Job drawing, mm, ordinate dimensions from the low corner. One solid piece. Coordinates: 2 decimals unless noted, no trailing zeros. Loops run counter-clockwise (first coordinate to the right, second up) from the corner with the lowest first, then second, coordinate; pieces in that order, holes last. Notation, with made-up numbers: (9, 22.25) -> (19, 22.25) arc R32 cw to (19, 49.25) -> close; hole circle Ø11 at (65, -31). An arc over 180 degrees is marked (long way). Use one line per item in the form item = value. Start each with the question number.
(1) Band-saw the part on C-C on y = 1.4. Give the cut face in (x, z).
(2) Band-saw the part on B-B on x = 17.7. Give the cut face in (y, z).
(3) Drill centre lines: L1, parallel to X at y = 1.55, z = 10.5; L2, parallel to Y at x = 16, z = 17.25; L3, parallel to X at y = 2.95, z = 11.5. Where is each one in solid material? Low to high. Write a range as [from, to].
(4) Pin check, flat tips, straight feed: P1, Ø1.8, axis at x = 10.5, z = 17.7, coming from the +Y side; P2, Ø1.5, axis at x = 7, y = 2.5, coming from the -Z side; P3, Ø2, axis at y = 4, z = 12.5, coming from the -X side. Stop position of each tip, or through.
(5) Mould opens along X. For the marked faces 1, 2 and 3 say: +X half, -X half, draft (parallel to the pull), parting line (faces both ways), or undercut.
(6) Band-saw the part on A-A on z = 10.5. Give the cut face in (x, y), then the cut area to 3 significant figures.
(7) Band-saw the part on D-D on z = 3.25. Give the cut face in (x, y), then the cut area to 3 significant figures.
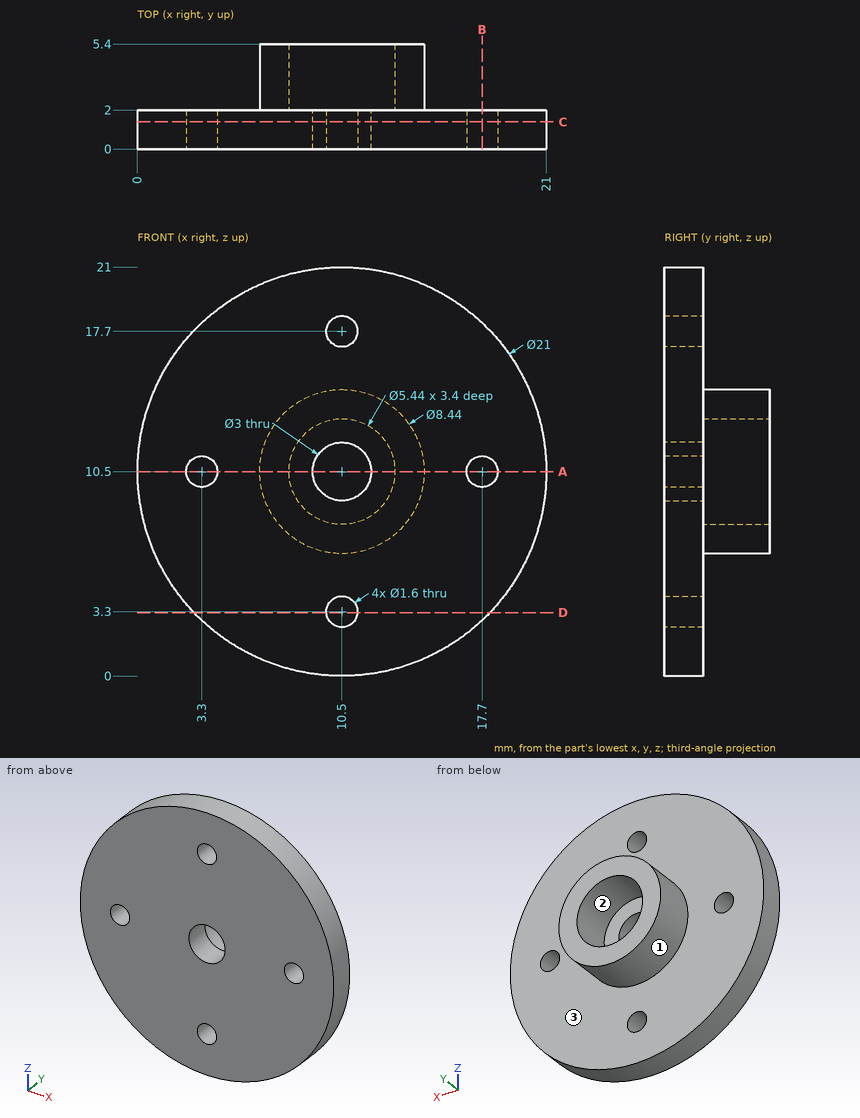
A:
q1.outline = circle Ø21 at (10.5, 10.5); hole circle Ø1.6 at (3.3, 10.5); hole circle Ø3 at (10.5, 10.5); hole circle Ø1.6 at (10.5, 3.3); hole circle Ø1.6 at (10.5, 17.7); hole circle Ø1.6 at (17.7, 10.5)
q2.outline = (0, 2.86) -> (2, 2.86) -> (2, 9.7) -> (0, 9.7) -> close; (0, 11.3) -> (2, 11.3) -> (2, 18.14) -> (0, 18.14) -> close
q3.L1 = [0, 2.5], [4.1, 9], [12, 16.9], [18.5, 21]
q3.L2 = [0, 2]
q3.L3 = [6.4, 7.97], [13.03, 14.6]
q4.P1 = 2
q4.P2 = 0.42
q4.P3 = 6.4
q5.face_1 = parting line
q5.face_2 = undercut
q5.face_3 = draft
q6.outline = (0, 0) -> (2.5, 0) -> (2.5, 2) -> (0, 2) -> close; (4.1, 0) -> (9, 0) -> (9, 2) -> (7.78, 2) -> (7.78, 5.4) -> (6.28, 5.4) -> (6.28, 2) -> (4.1, 2) -> close; (12, 0) -> (16.9, 0) -> (16.9, 2) -> (14.72, 2) -> (14.72, 5.4) -> (13.22, 5.4) -> (13.22, 2) -> (12, 2) -> close; (18.5, 0) -> (21, 0) -> (21, 2) -> (18.5, 2) -> close
q6.area = 39.8 mm²
q7.outline = (2.9, 0) -> (9.7, 0) -> (9.7, 2) -> (2.9, 2) -> close; (11.3, 0) -> (18.1, 0) -> (18.1, 2) -> (11.3, 2) -> close
q7.area = 27.2 mm²
